```python
from build123d import *

# Parameters (mm, degrees)
SKETCH4_R           = 16.9545
BOSS_EXTRUDE1_DEPTH = 45.72
SKETCH5_R           = 16.9545
BOSS_EXTRUDE2_DEPTH = 50.8
SKETCH9_R           = 16.9545
BOSS_EXTRUDE3_DEPTH = 45.72
SKETCH10_R          = 9.525
CUT_EXTRUDE1_DEPTH  = 12.7
SKETCH12_R          = 9.525
CUT_EXTRUDE2_DEPTH  = 12.7


with BuildPart() as part:
    # Sketch4 → Boss-Extrude1 (new body)
    with BuildSketch(Plane(origin=(0, 0, 0), x_dir=(0, 0, -1), z_dir=(1, 0, 0))):
        Circle(SKETCH4_R)
    extrude(amount=BOSS_EXTRUDE1_DEPTH)

    # Sketch5 → Boss-Extrude2 (add)
    with BuildSketch(Plane(origin=(45.72, 0, 0), x_dir=(0, 0, -1), z_dir=(0.906307787, -0.422618262, 0))):
        Circle(SKETCH5_R)
    extrude(amount=BOSS_EXTRUDE2_DEPTH)

    # Sketch9 → Boss-Extrude3 (add)
    with BuildSketch(Plane(origin=(91.760435581, -21.469007696, 0), x_dir=(0.766044443, 0.64278761, 0), z_dir=(-0.64278761, 0.766044443, 0))):
        Circle(SKETCH9_R)
    extrude(amount=-BOSS_EXTRUDE3_DEPTH)

    # Sketch10 → Cut-Extrude1 (cut)
    with BuildSketch(Plane(origin=(77.87287371, -92.805277009, 0), x_dir=(0.766044443, 0.64278761, 0), z_dir=(0.64278761, -0.766044443, 0))):
        with Locations((56.492559636, 0)):
            Circle(SKETCH10_R)
    extrude(amount=-CUT_EXTRUDE1_DEPTH, mode=Mode.SUBTRACT)

    # Sketch12 → Cut-Extrude2 (cut)
    with BuildSketch(Plane.ZY):
        Circle(SKETCH12_R)
    extrude(amount=-CUT_EXTRUDE2_DEPTH, mode=Mode.SUBTRACT)


solid = part.part
```
Design review of the part built by this model. Coordinates are the model's own, in mm. A direction names the side the tool comes from. Coordinates: 2 decimals unless noted, no trailing zeros. Order: outer loops, then holes, each group sorted by start corner. A loop starts at its lowest first (then second) coordinate and runs counter-clockwise, first axis right, second up. Notation, with made-up numbers: (64.25, 35) - (87.25, 35) arc R35 ccw to (87.25, 69) - close; hole circle Ø5 at (60.5, 32). An arc over 180 degrees is marked (long way). Answer in a Markdown table with one row per item.
(1) Consider section B-B on z = -11.5. State the section outline as (x, y) points.
Checked values:
| item | result |
|---|---|
| outline | (0, -12.46) - (42.96, -12.46) - (83.99, -31.59) - (111.61, -64.5) - (130.69, -48.48) - (101.3, -13.46) - (91.76, -21.47) - (97.03, -10.18) - (50.99, 11.29) - (45.72, 0) - (45.72, 12.46) - (0, 12.46) - close |
(2) For faces 1 (the flat face through (126.74, -51.8, 7.3)), 2 (the flat face through (112.88, -46.85, 0.13)), 3 (the cylindrical face through (22.54, 16.81, 2.21)), list the 3-axis set-ups (+Z, -Z, +X, -X, +Y, -Y) from which the entire face can be reached by the end or side of a thin tool; tool diameter is ignored.
Checked values:
| item | result |
|---|---|
| face 1 | +Z, -Z, +X, -Y |
| face 2 | none |
| face 3 | -X |
(3) Consider section C-C on z = -2. State the section outline as (x, y) points, plus the area to 3 significant figures.
Checked values:
| item | result |
|---|---|
| outline | (0, -16.84) - (41.99, -16.84) - (81.26, -35.15) - (108.25, -67.31) - (114.01, -62.48) - (105.85, -52.75) - (120.12, -40.78) - (128.28, -50.51) - (134.05, -45.67) - (104.66, -10.65) - (91.76, -21.47) - (98.88, -6.21) - (52.84, 15.26) - (45.72, 0) - (45.72, 16.84) - (0, 16.84) - (0, 9.31) - (12.7, 9.31) - (12.7, -9.31) - (0, -9.31) - close |
| area | 4,190 mm^2 |
(4) Clearance check with flat-ended pins moving along their axes: pin 1 (4 mm diameter, centred on y = -50, z = -8, fed in from -X); pin 2 (5 mm diameter, centred on x = 82.5, z = 8, fed in from -Y); pin 3 (8 mm diameter, centred on y = -17.5, z = -12.5, fed in from +X). State where each tip first meets the part, or that it passes through.
Checked values:
| item | result |
|---|---|
| pin 1 | x = 94.08 |
| pin 2 | y = -37.21 |
| pin 3 | x = 108.98 |
(5) Consider section A-A on z = 15. State the section outline as (x, y) points.
Checked values:
| item | result |
|---|---|
| outline | (0, -7.9) - (43.97, -7.9) - (86.83, -27.89) - (115.09, -61.57) - (127.2, -51.41) - (97.81, -16.39) - (91.76, -21.47) - (95.1, -14.31) - (49.06, 7.16) - (45.72, 0) - (45.72, 7.9) - (0, 7.9) - close |
(6) Wall thickness on line 1 along Y through (x, z) = (8.75, 0) (1 decimal); line 2 along X through (y, z) = (2, 0); line 3 along Y through (x, z) = (95.5, 8.5): over which ranges is each line inside the solid? List them lowest first. Write a range as from..to.
Checked values:
| item | result |
|---|---|
| line 1 | -17..-9.5, 9.5..17 |
| line 2 | 12.7..45.72, 46.65..81.55 |
| line 3 | -48.75..-18.33, -13.45..-7.03 |
(7) The part is to be moulded in two halves that separate along X. For faces 4 (the cylindrical face through (6.261, -5.796, -7.559)), 5 (the flat face through (0, -7, -7)), 6 (the flat face through (94.597, -15.386, 0.237)), say which applies: released by +X, released by -X, zero draft, split by the parting line, or undercut.
Checked values:
| item | result |
|---|---|
| face 4 | zero draft |
| face 5 | released by -X |
| face 6 | undercut |
